Source: CAD feature listing. Evaluate the final solid. Frame: model axes, mm. A direction names the side the tool comes from. Give positions to 0.01 mm unless a question says otherwise; leave off trailing zeros. Write each loop counter-clockwise with the first axis right and the second up, starting at its lowest first coordinate (ties: lowest second). Pieces come first, ordered by that corner, then holes. Notation, with made-up numbers: (35.5, 3.25) -> (54.5, 3.25) arc R16 cw to (54.5, 30.25) -> close; hole circle Ø8 at (14, -17.5). An arc over 180 degrees is marked (long way). Answer as a JSON object with one key per item and string values. Group by question number.
Item 1: Section query B-B on y = 18.5. Return the cut outline in (x, z), plus the area to 3 significant figures.
Item 2: Access query for faces 1 (the face through (-32.275, 3, 13)), 2 (the face through (-54.68, 22.61, -18.65)), 3 (the face through (-38.275, 1, -22)). Directions: +Z, -Z, +X, -X, +Y, -Y. A direction counts if a zero-diameter tool reaches every point of the face in a straight line with its end or side. Return the directions, or none.
Item 3: Section query D-D on x = -86. Return the cut outline in (y, z).
Item 4: Ray query, probe 1 along Y at (x, z) = (-1, -14.5); probe 2 along Z at (x, y) = (-109, 2); probe 3 along X at (y, z) = (36, -11). Return the intervals inside material, ascending. Write a range as from..to.
Item 5: Section query C-C on z = 10. Return the cut outline in (x, y).
Item 6: Section query A-A on x = 5.5. Return the cut outline in (y, z), plus the area to 3 significant figures.
Item 7: First-contact query: pin 1 Ø3 at (x, z) = (-33, -14.5) entering from +Y; pin 2 Ø1.4 at (x, y) = (-72, 7.5) entering from +Z; pin 3 Ø1.8 at (x, y) = (-13, 2) entering from -Z; pin 4 Ø1.5 at (x, y) = (-52.5, 7.5) entering from -Z. Flat tips, straight axial feed; report the tip coordinate or a pass-through.
Item 8: Pull-direction query (Y, two-part tool) for faces 4 (the face through (-73, 6, -2)), 5 (the face through (-107.764, 4.798, -23.368)), 6 (the face through (-36.588, 3, -20)); classes: pulls with the +Y half, pulls with the -Y half, needs draft (parallel to the pull), parting line crosses it, or undercut.
from build123d import *

# Parameters (mm, degrees)
SKETCH1_W            = 37.613618603
SKETCH1_H            = 47.017023253
SKETCH1_W_2          = 37.613618602
BOSS_EXTRUDE1_DEPTH  = 6
BOSS_EXTRUDE2_DEPTH  = 6
MIRROR3_COPY_1_DEPTH = 6
SKETCH6_W            = 8.533488923
SKETCH6_H            = 15.820834786
CUT_EXTRUDE2_DEPTH   = 2
SKETCH7_W            = 8.533488923
SKETCH7_H            = 10.900786406
CUT_EXTRUDE3_DEPTH   = 16
BOSS_EXTRUDE6_DEPTH  = 4
SKETCH9_W            = 9.784219632
SKETCH9_H            = 16.89117049
CUT_EXTRUDE4_DEPTH   = 2
SKETCH10_W           = 9.784219632
SKETCH10_H           = 11.02968992
CUT_EXTRUDE5_DEPTH   = 15
BOSS_EXTRUDE8_DEPTH  = 0.7
BOSS_EXTRUDE9_DEPTH  = 0.7
SKETCH15_W           = 7.842146402
SKETCH15_H           = 8.765171011
BOSS_EXTRUDE11_DEPTH = 0.7
BOSS_EXTRUDE12_DEPTH = 0.7
BOSS_EXTRUDE13_DEPTH = 0.7
BOSS_EXTRUDE15_DEPTH = 6
BOSS_EXTRUDE16_DEPTH = 1
SKETCH25_R           = 0.785617121
BOSS_EXTRUDE17_DEPTH = 13
BOSS_EXTRUDE18_DEPTH = 1
SKETCH27_R           = 0.813635411
BOSS_EXTRUDE19_DEPTH = 12


with BuildPart() as part:
    # Sketch1 → Boss-Extrude1 (new body)
    with BuildSketch(Plane(origin=(0, 0, 0), x_dir=(1, 0, 0), z_dir=(0, 1, 0))):
        Polygon((-163.115635978, 16.680412456), (-163.115635978, -40.614150466), (-163.115635978, -42.336610797), (17.338838432, -42.336610797), (17.338838432, 16.680412456), (16.48228959, 16.680412456), align=None)
        with Locations((-138.308826677, -12.82809917)):
            Rectangle(SKETCH1_W, SKETCH1_H, mode=Mode.SUBTRACT)
        with Locations((-94.695208074, -12.82809917)):
            Rectangle(SKETCH1_W_2, SKETCH1_H, mode=Mode.SUBTRACT)
        with Locations((-51.081589472, -12.82809917)):
            Rectangle(SKETCH1_W, SKETCH1_H, mode=Mode.SUBTRACT)
        with Locations((-7.467970869, -12.82809917)):
            Rectangle(SKETCH1_W_2, SKETCH1_H, mode=Mode.SUBTRACT)
    extrude(amount=BOSS_EXTRUDE1_DEPTH)

    # Sketch2 → Boss-Extrude2 (add)
    with BuildSketch(Plane.ZY.offset(119.502017375)):
        Polygon((-10.680412456, 6), (-10.680412456, 7.806965874), (-20.737358395, 7.806965874), (-25.925828115, 1.87209116), (-25.925828115, -3.073895358), (-25.925828115, -6.20063921), (-20.737358395, 0), (-16.680412456, 0), (-10.680412456, 0), align=None)
    boss_extrude2 = extrude(amount=-BOSS_EXTRUDE2_DEPTH)

    # Mirror2: Boss-Extrude2 across plane
    add(boss_extrude2.mirror(Plane(origin=(-75.888398773, 6, -10.680412456), x_dir=(0, 0, 1), z_dir=(-1, 0, 0))))

    # Mirror3 copy 1 sketch → Mirror3 copy 1 (add)
    with BuildSketch(Plane.ZY.offset(32.27478017)):
        Polygon((-10.680412456, 6), (-10.680412456, 7.806965874), (-20.737358395, 7.806965874), (-25.925828115, 1.87209116), (-25.925828115, -3.073895358), (-25.925828115, -6.20063921), (-20.737358395, 0), (-16.680412456, 0), (-10.680412456, 0), align=None)
    extrude(amount=-MIRROR3_COPY_1_DEPTH)

    # Mirror4: Boss-Extrude2 across plane
    add(boss_extrude2.mirror(Plane.ZY.offset(113.502017375)))

    # Sketch6 → Cut-Extrude2 (cut)
    with BuildSketch(Plane(origin=(0, 7.806965874, 0), x_dir=(1, 0, 0), z_dir=(0, 1, 0))):
        with Locations((-32.321100626, 18.590829849)):
            Rectangle(SKETCH6_W, SKETCH6_H)
    extrude(amount=-CUT_EXTRUDE2_DEPTH, mode=Mode.SUBTRACT)

    # Sketch7 → Cut-Extrude3 (cut)
    with BuildSketch(Plane(origin=(0, 5.806965874, 0), x_dir=(1, 0, 0), z_dir=(0, 1, 0))):
        with Locations((-32.321100626, 22.033512706)):
            Rectangle(SKETCH7_W, SKETCH7_H)
    extrude(amount=-CUT_EXTRUDE3_DEPTH, mode=Mode.SUBTRACT)

    # Sketch8 → Boss-Extrude6 (add)
    with BuildSketch(Plane(origin=(0, 0, -16.680412456), x_dir=(-1, 0, 0), z_dir=(0, 0, -1))):
        Polygon((38.27478017, 4.522273807), (38.27478017, 8.450147148), (69.772707479, 38.666586062), (69.772707479, 48.334730149), (70.874011488, 48.334730149), (70.874011488, 37.278255422), (69.772707479, 37.278255422), (39.158061482, 7.529405606), (39.158061482, 4.522273807), align=None)
    boss_extrude6 = extrude(amount=BOSS_EXTRUDE6_DEPTH)

    # Sketch9 → Cut-Extrude4 (cut)
    with BuildSketch(Plane(origin=(0, 7.806965874, 0), x_dir=(1, 0, 0), z_dir=(0, 1, 0))):
        with Locations((-113.591226463, 19.125997701)):
            Rectangle(SKETCH9_W, SKETCH9_H)
    extrude(amount=-CUT_EXTRUDE4_DEPTH, mode=Mode.SUBTRACT)

    # Sketch10 → Cut-Extrude5 (cut)
    with BuildSketch(Plane(origin=(0, 5.806965874, 0), x_dir=(1, 0, 0), z_dir=(0, 1, 0))):
        with Locations((-113.591226463, 22.097964463)):
            Rectangle(SKETCH10_W, SKETCH10_H)
    extrude(amount=-CUT_EXTRUDE5_DEPTH, mode=Mode.SUBTRACT)

    # Mirror7: Boss-Extrude6 across plane
    add(boss_extrude6.mirror(Plane(origin=(-72.533385445, 0, 0), x_dir=(0, 0, 1), z_dir=(1, 0, 0))))

    # Sketch12 → Boss-Extrude8 (add)
    with BuildSketch(Plane(origin=(-107.502017375, 0, 0), x_dir=(0, 0, -1), z_dir=(1, 0, 0))):
        Polygon((16.680412456, 6), (16.680412456, 0), (20.737358395, 0), (25.925828115, -6.20063921), (25.925828115, 1.87209116), (20.737358395, 7.806965874), (10.680412456, 7.806965874), (10.680412456, 6), align=None)
    extrude(amount=BOSS_EXTRUDE8_DEPTH)

    # Sketch14 → Boss-Extrude9 (add)
    with BuildSketch(Plane(origin=(-118.483336279, 0, 0), x_dir=(0, 0, -1), z_dir=(1, 0, 0))):
        Polygon((16.583119503, 0), (16.583119503, 5.806965874), (10.680412456, 5.806965874), (10.680412456, 7.806965874), (20.737358395, 7.806965874), (25.925828115, 1.87209116), (25.925828115, -6.20063921), (20.737358395, 0), align=None)
    extrude(amount=BOSS_EXTRUDE9_DEPTH)

    # Sketch15 → Boss-Extrude11 (add)
    with BuildSketch(Plane.ZY.offset(70.874011488)):
        with Locations((-20.601485657, 43.952144644)):
            Rectangle(SKETCH15_W, SKETCH15_H)
    extrude(amount=BOSS_EXTRUDE11_DEPTH)

    # Sketch19 → Boss-Extrude12 (add)
    with BuildSketch(Plane(origin=(-74.192759403, 0, 0), x_dir=(0, 0, -1), z_dir=(1, 0, 0))):
        Polygon((20.680412456, 48.334730149), (20.754843595, 39.792896823), (16.566782326, 39.792896823), (16.680412456, 48.334730149), align=None)
    extrude(amount=BOSS_EXTRUDE12_DEPTH)

    # Sketch21 → Boss-Extrude13 (add)
    with BuildSketch(Plane(origin=(-74.192759403, 0, 0), x_dir=(0, 0, -1), z_dir=(1, 0, 0))):
        Polygon((20.754843595, 39.792896823), (24.537534544, 39.792896823), (24.537534544, 48.362951427), (20.680412456, 48.334730149), align=None)
    extrude(amount=BOSS_EXTRUDE13_DEPTH)

    # Sketch23 → Boss-Extrude15 (add)
    with BuildSketch(Plane.ZY.offset(75.888398773)):
        Polygon((36.336610797, 6), (36.336610797, 7.794899668), (-15.54173244, 38.987033262), (-15.54173244, 42.801373137), (-17.017265085, 42.801373137), (-17.017265085, 38.335404827), (-17.017265085, 36.955229626), (31.491887766, 7.794899668), (31.491887766, 4.688712486), (36.336610797, 4.688712486), align=None)
    extrude(amount=-BOSS_EXTRUDE15_DEPTH)

    # Sketch24 → Boss-Extrude16 (add)
    with BuildSketch(Plane.ZY.offset(119.502017375)):
        Polygon((-22.278203382, -0.491017032), (-23.054410428, 0.85341301), (-24.606824521, 0.85341301), (-25.383031568, -0.491017032), (-24.606824521, -1.835447074), (-23.054410428, -1.835447074), align=None)
    extrude(amount=BOSS_EXTRUDE16_DEPTH)

    # Sketch25 → Boss-Extrude17 (add)
    with BuildSketch(Plane(origin=(-106.802017375, 0, 0), x_dir=(0, 0, -1), z_dir=(1, 0, 0))):
        with Locations((24.059849536, -0.571927467)):
            Circle(SKETCH25_R)
    extrude(amount=-BOSS_EXTRUDE17_DEPTH)

    # Sketch26 → Boss-Extrude18 (add)
    with BuildSketch(Plane(origin=(-26.27478017, 0, 0), x_dir=(0, 0, -1), z_dir=(1, 0, 0))):
        Polygon((25.53835309, 0), (24.736565321, 1.388737154), (23.132989782, 1.388737154), (22.331202013, 0), (23.132989782, -1.388737154), (24.736565321, -1.388737154), align=None)
    extrude(amount=BOSS_EXTRUDE18_DEPTH)

    # Sketch27 → Boss-Extrude19 (add)
    with BuildSketch(Plane.ZY.offset(38.27478017)):
        with Locations((-23.747895792, -0.52869674)):
            Circle(SKETCH27_R)
    extrude(amount=-BOSS_EXTRUDE19_DEPTH)


solid = part.part
Worked answers:
{
 "1": {"outline": "(-96.32, -20.68) -> (-94.62, -20.68) -> (-94.62, -16.68) -> (-96.32, -16.68) -> close; (-75.89, 13.68) -> (-69.89, 13.68) -> (-69.89, 18.53) -> (-75.89, 18.53) -> close; (-50.45, -20.68) -> (-48.75, -20.68) -> (-48.75, -16.68) -> (-50.45, -16.68) -> close", "area": "42.7 mm^2"},
 "2": {"face 1": "+Y, -Y", "face 2": "+Z, -Z, -Y", "face 3": "-Z, -Y"},
 "3": {"outline": "(0, -16.68) -> (6, -16.68) -> (6, -10.68) -> (0, -10.68) -> close; (0, 36.34) -> (6, 36.34) -> (6, 42.34) -> (0, 42.34) -> close; (26.88, -20.68) -> (28.4, -20.68) -> (28.4, -16.68) -> (26.88, -16.68) -> close"},
 "4": {"probe 1": "0..6", "probe 2": "-16.58..-10.68, 36.34..42.34", "probe 3": "-75.89..-69.89"},
 "5": {"outline": "(-163.12, 0) -> (-157.12, 0) -> (-157.12, 6) -> (-163.12, 6) -> close; (-119.5, 0) -> (-113.5, 0) -> (-113.5, 6) -> (-119.5, 6) -> close; (-75.89, 0) -> (-69.89, 0) -> (-69.89, 6) -> (-75.89, 6) -> close; (-75.89, 20.71) -> (-69.89, 20.71) -> (-69.89, 23.63) -> (-75.89, 23.63) -> close; (-32.27, 0) -> (-26.27, 0) -> (-26.27, 6) -> (-32.27, 6) -> close; (11.34, 0) -> (17.34, 0) -> (17.34, 6) -> (11.34, 6) -> close"},
 "6": {"outline": "(0, -16.68) -> (6, -16.68) -> (6, -10.68) -> (0, -10.68) -> close; (0, 36.34) -> (6, 36.34) -> (6, 42.34) -> (0, 42.34) -> close", "area": "72.0 mm^2"},
 "7": {"pin 1": "y = 5.81", "pin 2": "z = 36.34", "pin 3": "z = -16.68", "pin 4": "through"},
 "8": {"face 4": "undercut", "face 5": "pulls with the +Y half", "face 6": "needs draft"}
}
